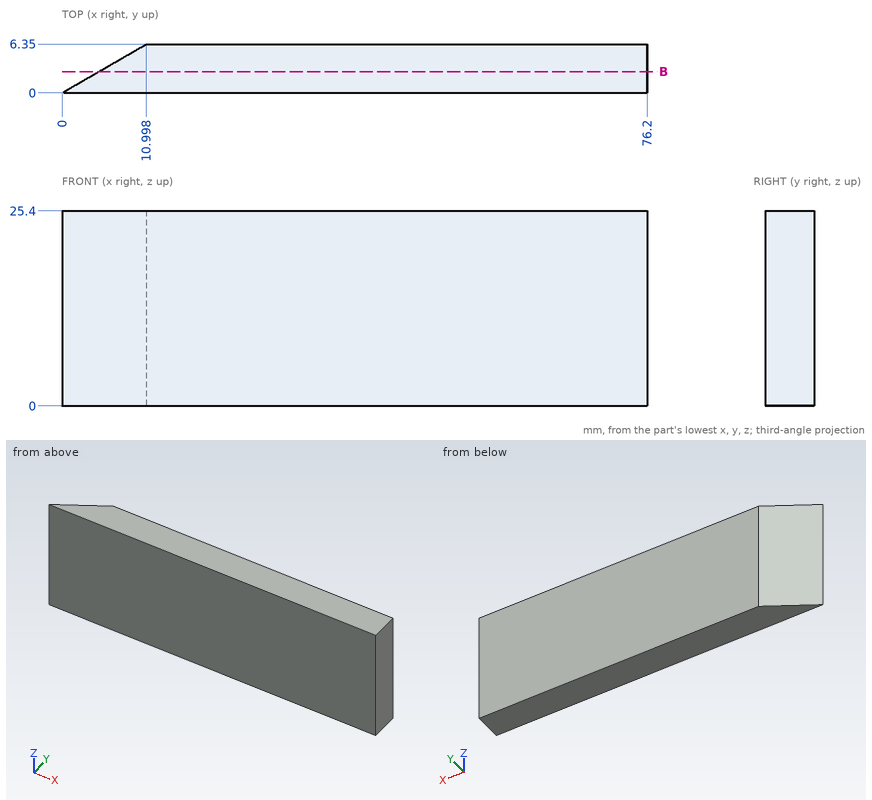
Geometry: see drawing. Coordinates: mm, zero at the bounding-box minimum. Round coordinates to 2 decimals unless told otherwise and drop trailing zeros. Write each loop counter-clockwise with the first axis right and the second up, starting at its lowest first coordinate (ties: lowest second). Pieces come first, ordered by that corner, then holes. Notation, with made-up numbers: (22.5, 4) -> (70.5, 4) arc R15 ccw to (70.5, 33) -> close; hole circle Ø10 at (41, 86). An arc over 180 degrees is marked (long way). Answer as CSV lines item,"result".
1. Contact query for flat-ended pins moving along their axis: P1, Ø12, axis at x = 66.5, z = 21.5, coming from the -Y side; P2, Ø1.5, axis at y = 3.5, z = 11, coming from the -X side (1 decimal). Output: stop coordinate, or through.
Geometry says:
P1,"stops at y = 0"
P2,"stops at x = 4.8"
2. Section B-B (y = 2.75). Return the cut outline in (x, z), plus the area to 3 significant figures.
Geometry says:
outline,"(4.76, 0) -> (76.2, 0) -> (76.2, 25.4) -> (4.76, 25.4) -> close"
area,"1,810 mm^2"
3. Ray query, L1, parallel to Y at x = 3, z = 22.25; L2, parallel to X at y = 1.25, z = 1.5 (1 decimal); L3, parallel to X at y = 2, z = 11.5 (1 decimal). Return the intervals inside material, ascending. Write a range as [from, to].
Geometry says:
L1,"y = [0, 1.73]"
L2,"x = [2.2, 76.2]"
L3,"x = [3.5, 76.2]"
